Can you work these out from the model? Positions are in its coordinate system, mm. Face numbers are marked on the shaded views. A direction names the side the tool comes from. Coordinates: 2 decimals unless noted, no trailing zeros. Order: outer loops, then holes, each group sorted by start corner. A loop starts at its lowest first (then second) coordinate and runs counter-clockwise, first axis right, second up. Notation, with made-up numbers: (43, -34.5) -> (50, -34.5) arc R25 cw to (50, 4.5) -> close; hole circle Ø9 at (81.25, 72). An arc over 180 degrees is marked (long way). Use a Markdown table: item, result. Add a question column.
1. If I drill on line 1 along X through (y, z) = (2, 17); line 2 along Z through (x, y) = (-0.5, 4.25); line 3 along X through (y, z) = (8.25, 15), over which ranges is the centre line in solid material (lowest first)? Write a range as from..to.
2. For pin 1 Ø1.8 at (x, y) = (14.5, 7) entering from +Z; pin 2 Ø2.5 at (x, z) = (-37.5, 0.5) entering from +Y; pin 3 Ø6 at (x, z) = (8.5, -0.5) entering from +Y, each with a flat end and sliding along its axis, tell me the tip position at first contact or that it passes through.
3. Suppose I cut it at B-B, the plane x = -33. List the corners of the cut face in (y, z) for me, then the cut area to 3 significant figures.
4. Suppose I cut it at A-A, the plane z = 17. List the corners of the cut face in (x, y) for me.
5. We'd pull the mould along X, two halves only. Please class the marked faces 1, 2 and 3: pulls with the +X half, pulls with the -X half, needs draft (parallel to the pull), parting line crosses it, or undercut.
6. Suppose I cut it at D-D, the plane y = 9.25. List the corners of the cut face in (x, z) for me.
7. For the marked faces 4, 5, 6, 7 and 8, which set-ups out of +Z, -Z, +X, -X, +Y, -Y let a thin tool reach every point of the face, with its end or its side?
8. Suppose I cut it at C-C, the plane z = 0. List the corners of the cut face in (x, y) for me, then the cut area to 3 significant figures.
```python
from build123d import *

# Parameters (mm, degrees)
BOSS_EXTRUDE1_DEPTH       = 10
SKETCH2_R                 = 3.5
CUT_EXTRUDE1_DEPTH        = 10
CUT_EXTRUDE2_DEPTH        = 78.491935064
FILLET1_R                 = 2
MOVE_START                = 7.5
MOVE_FACE1_DEPTH          = 2.5
USB_C_CHARGE_ACCESS_DEPTH = 5
FILLET3_R                 = 2


# Read off the part's stored shape, not the designer's step: Move Face1
with BuildPart() as part:
    # Sketch1 → Boss-Extrude1 (new body)
    with BuildSketch(Plane(origin=(0, 0, 0), x_dir=(1, 0, 0), z_dir=(0, 1, 0))):
        Polygon((20, -10), (10, -10), (10, -24), (-10, -24), (-10, -10), (-23, -10), (-23, -24), (-43, -24), (-43, -10), (-53, -10), (-53, 10), (20, 10), align=None)
    extrude(amount=BOSS_EXTRUDE1_DEPTH)

    # Sketch2 → Cut-Extrude1 (cut)
    with BuildSketch(Plane(origin=(0, 10, 0), x_dir=(1, 0, 0), z_dir=(0, 1, 0))):
        with Locations(Location((0, -17, 0), (0, 0, 270))):
            Circle(SKETCH2_R)
        with Locations(Location((-33, -17, 0), (0, 0, 270))):
            Circle(SKETCH2_R)
    extrude(amount=-CUT_EXTRUDE1_DEPTH, mode=Mode.SUBTRACT)

    # Sketch3 → Cut-Extrude2 (cut, through all)
    with BuildSketch(Plane(origin=(20, 0, 0), x_dir=(0, 0, -1), z_dir=(1, 0, 0))):
        with BuildLine():
            Line((-2.692582404, 3), (2.692582404, 3))
            ThreePointArc((2.692582404, 3), (0, 17.5), (-2.692582404, 3))
        make_face()
    extrude(amount=-CUT_EXTRUDE2_DEPTH, mode=Mode.SUBTRACT)

    # Fillet1
    fillet1_edges = [part.edges().sort_by_distance(p)[0] for p in [
        (-16.5, 0, -10),
        (20, 5, 10),
        (10, 5, 10),
        (10, 5, 24),
        (-10, 5, 24),
        (-10, 5, 10),
        (-23, 5, 10),
        (-23, 5, 24),
        (-43, 5, 24),
        (-43, 5, 10),
        (-53, 5, 10),
        (-53, 5, -10),
        (20, 5, -10),
    ]]
    fillet(fillet1_edges, radius=FILLET1_R)

    # Move Face1 outline → Move Face1 (cut)
    with BuildSketch(Plane(origin=(0, 0, 0), x_dir=(1, 0, 0), z_dir=(0, 1, 0)).offset(MOVE_START)):
        with BuildLine():
            Line((18, 10), (-51, 10))
            ThreePointArc((-51, 10), (-52.414213562, 9.414213562), (-53, 8))
            Line((-53, 8), (-53.000000001, 6))
            Line((-53.000000001, 6), (20.000000001, 6))
            Line((20.000000001, 6), (20, 8))
            ThreePointArc((20, 8), (19.414213562, 9.414213562), (18, 10))
        make_face()
    extrude(amount=MOVE_FACE1_DEPTH, mode=Mode.SUBTRACT)

    # Sketch4 → USB-C charge access (cut, symmetric)
    with BuildSketch(Plane(origin=(0, 3, 0), x_dir=(1, 0, 0), z_dir=(0, 1, 0))):
        with BuildLine():
            Line((-10, -3.75), (-23, -3.75))
            ThreePointArc((-23, -3.75), (-26.75, 0), (-23, 3.75))
            Line((-23, 3.75), (-10, 3.75))
            ThreePointArc((-10, 3.75), (-6.25, 0), (-10, -3.75))
        make_face()
    extrude(amount=USB_C_CHARGE_ACCESS_DEPTH, both=True, mode=Mode.SUBTRACT)

    # Fillet3
    fillet3_edges = [part.edges().sort_by_distance(p)[0] for p in [
        (-16.5, 0, 3.75),
        (-16.5, 0, -3.75),
        (-6.25, 0, 0),
        (-26.75, 0, 0),
    ]]
    fillet(fillet3_edges, radius=FILLET3_R)


solid = part.part
```
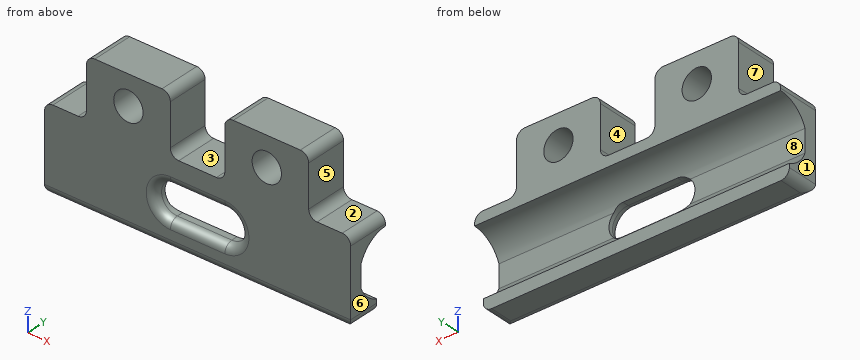
Worked out:
| question | item | result |
|---|---|---|
| 1 | line 1 | x = -43..-36.5, -29.5..-23, -10..-3.5, 3.5..10 |
| 1 | line 2 | z = -10..-4.82, 4.82..13.54, 20.46..24 |
| 1 | line 3 | x = -43..-35.87, -30.13..-23, -10..-2.87, 2.87..10 |
| 2 | pin 1 | stops at z = 10 |
| 2 | pin 2 | stops at y = 3 |
| 2 | pin 3 | stops at y = 3.37 |
| 3 | outline | (0, -8) arc R2 ccw to (2, -10) -> (7.5, -10) -> (7.5, -7.07) arc R7.5 cw to (3, -2.69) -> (3, 2.69) arc R7.5 cw to (10, 7.5) -> (10, 13.5) -> (0, 13.5) -> close; (0, 20.5) -> (10, 20.5) -> (10, 24) -> (0, 24) -> close |
| 3 | area | 176 mm² |
| 4 | outline | (-43, 0) -> (-36.5, 0) -> (-36.5, 10) -> (-43, 10) -> close; (-29.5, 0) -> (-23, 0) -> (-23, 10) -> (-29.5, 10) -> close; (-10, 0) -> (-3.5, 0) -> (-3.5, 10) -> (-10, 10) -> close; (3.5, 0) -> (10, 0) -> (10, 10) -> (3.5, 10) -> close |
| 5 | face 1 | pulls with the -X half |
| 5 | face 2 | needs draft |
| 5 | face 3 | undercut |
| 6 | outline | (-53, 7.46) -> (20, 7.46) -> (20, 8) arc R2 ccw to (18, 10) -> (12, 10) arc R2 cw to (10, 12) -> (10, 22) arc R2 ccw to (8, 24) -> (-8, 24) arc R2 ccw to (-10, 22) -> (-10, 12) arc R2 cw to (-12, 10) -> (-21, 10) arc R2 cw to (-23, 12) -> (-23, 22) arc R2 ccw to (-25, 24) -> (-41, 24) arc R2 ccw to (-43, 22) -> (-43, 12) arc R2 cw to (-45, 10) -> (-51, 10) arc R2 ccw to (-53, 8) -> close; hole circle Ø7 at (-33, 17); hole circle Ø7 at (0, 17) |
| 7 | face 4 | +Z, +Y, -Y |
| 7 | face 5 | +Z, +X, +Y, -Y |
| 7 | face 6 | +Z, -Z, +X, +Y, -Y |
| 7 | face 7 | +Z, -X, +Y, -Y |
| 7 | face 8 | +X, -X, +Y |
| 8 | outline | (-53, 0) -> (-28.75, 0) arc R2 ccw to (-26.75, 2) -> (-26.75, 3) -> (-53, 3) -> close; (-6.25, 2) arc R2 ccw to (-4.25, 0) -> (20, 0) -> (20, 3) -> (-6.25, 3) -> close |
| 8 | area | 156 mm² |
